from build123d import *

# Parameters (mm, degrees)
BOSS_EXTRUDE2_DEPTH = 1200
CUT_EXTRUDE2_DEPTH  = 1200


with BuildPart() as part:
    # Sketch4 → Boss-Extrude2 (new body)
    with BuildSketch(Plane(origin=(0, 0, 0), x_dir=(0, 0, -1), z_dir=(1, 0, 0))):
        with BuildLine():
            Line((-418.085663079, -116.728740424), (-167.287455413, -116.728740424))
            ThreePointArc((-167.287455413, -116.728740424), (-65.293961038, -84.661970634), (0, 0))
            Line((0, 0), (-17.8, 35))
            ThreePointArc((-17.8, 35), (-86.57752002, -49.822987688), (-191.015585124, -81.728740424))
            Line((-191.015585124, -81.728740424), (-418.085663079, -81.728740424))
            Line((-418.085663079, -81.728740424), (-913.455403633, -81.728740424))
            Line((-913.455403633, -81.728740424), (-913.455403633, -116.728740424))
            Line((-913.455403633, -116.728740424), (-418.085663079, -116.728740424))
        make_face()
    extrude(amount=BOSS_EXTRUDE2_DEPTH)

    # Sketch5 → Cut-Extrude2 (cut)
    with BuildSketch(Plane(origin=(0, -81.728740424, 0), x_dir=(1, 0, 0), z_dir=(0, 1, 0))):
        Polygon((0, -913.455403633), (450, -913.455403633), (0, -191.015585124), align=None)
        Polygon((1200, -191.015585124), (750, -913.455403633), (1200, -913.455403633), align=None)
    extrude(amount=-CUT_EXTRUDE2_DEPTH, mode=Mode.SUBTRACT)


solid = part.part
Design review of the part built by this model. Coordinates are the model's own, in mm. A direction names the side the tool comes from. Round coordinates to 2 decimals unless told otherwise and drop trailing zeros. Order: outer loops, then holes, each group sorted by start corner. A loop starts at its lowest first (then second) coordinate and runs counter-clockwise, first axis right, second up.
1) Consider section B-B (z = 221). State the section outline as (x, y) points.
The answers:
outline: (18.68, -116.73) - (1181.32, -116.73) - (1181.32, -81.73) - (18.68, -81.73) - close
2) Consider section D-D (x = 1064). State the section outline as (y, z) points.
The answers:
outline: (-116.73, 167.29) arc R178.24 ccw to (0, 0) - (35, 17.8) arc R186.88 cw to (-81.73, 191.02) - (-81.73, 409.35) - (-116.73, 409.35) - close
3) Clearance check with flat-ended pins moving along their axes: pin 1 Ø6 at (x, z) = (657, 147) entering from -Y; pin 2 Ø1 at (y, z) = (-92.5, 255) entering from +X; pin 3 Ø12 at (x, y) = (1056.5, -18.5) entering from +Z. State where each tip first meets the part, or that it passes through.
The answers:
pin 1: stops at y = -115.89
pin 2: stops at x = 1160.46
pin 3: stops at z = 56.42
4) Consider section C-C (y = 13.5). State the section outline as (x, z) points, plus the area to 3 significant figures.
The answers:
outline: (0, 6.87) - (1200, 6.87) - (1200, 28.15) - (0, 28.15) - close
area: 25,500 mm2
5) For L1, parallel to Y at x = 571, z = 634; L2, parallel to Z at x = 314.5, y = -48.5; L3, parallel to Z at x = 897.5, y = 6.5, list the stretches that pass through material, from the lowest coordinate up.
The answers:
L1: y = -116.73 to -81.73
L2: z = 27.05 to 84.64
L3: z = 3.31 to 32.29
6) Machinability: for faces 1 (the flat face through (978.15, -98.98, 547.18)), 2 (the flat face through (592, -81.729, 467)), which of the approach directions +Z, -Z, +X, -X, +Y, -Y give a long, thin tool a straight path to every point of the face, cutting with its end or side? Answer none if there is none.
The answers:
face 1: +Z, +X, +Y, -Y
face 2: +Z, +X, -X, +Y
7) Consider section A-A (x = 502.5). State the section outline as (y, z) points.
The answers:
outline: (-116.73, 167.29) arc R178.24 ccw to (0, 0) - (35, 17.8) arc R186.88 cw to (-81.73, 191.02) - (-81.73, 913.46) - (-116.73, 913.46) - close
